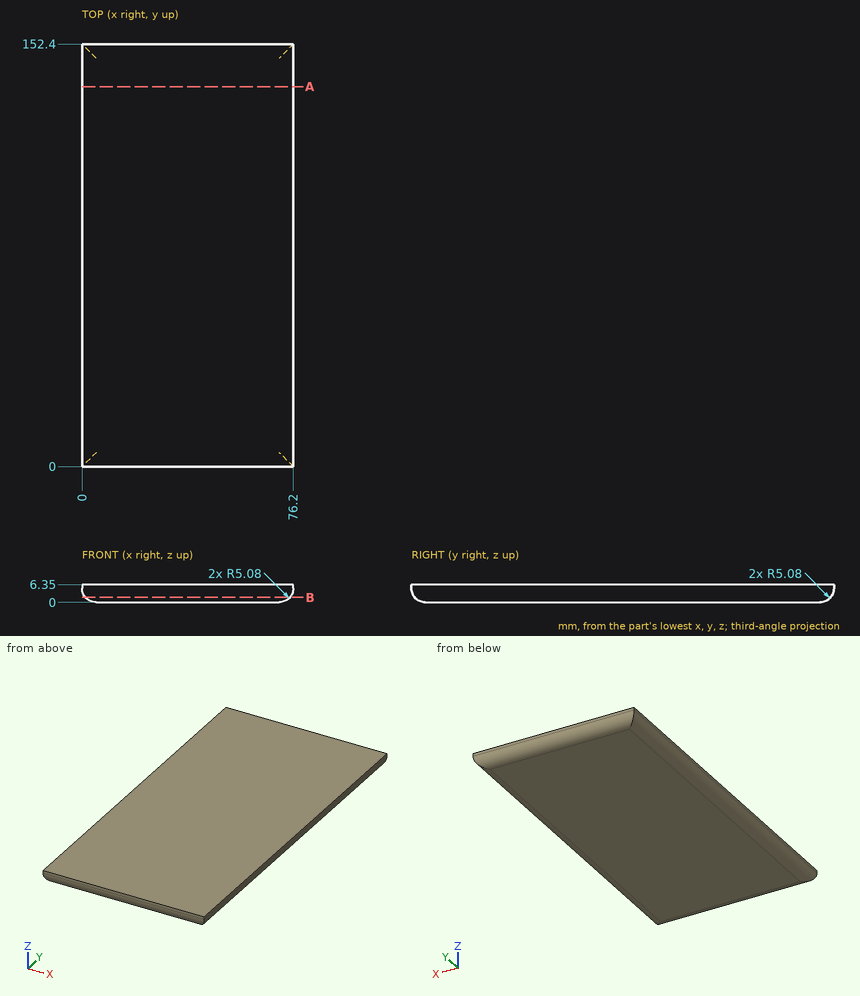
Source: three-view drawing plus pictorial views. Frame: mm from the lowest corner of the part. Give positions to 0.01 mm unless a question says otherwise; leave off trailing zeros. Write each loop counter-clockwise with the first axis right and the second up, starting at its lowest first coordinate (ties: lowest second). Pieces come first, ordered by that corner, then holes. Notation, with made-up numbers: (10.25, -36.75) -> (61.25, -36.75) arc R16 cw to (61.25, -27.75) -> close; hole circle Ø8 at (22, 23). An arc over 180 degrees is marked (long way). Answer in a Markdown table with one row per item.
(1) Pin query (flat end, axial travel): pin 1 (8 mm diameter, centred on x = 8.5, y = 16.5, fed in from -Z); pin 2 (1.5 mm diameter, centred on x = 56.5, z = 4, fed in from -Y). Return the tip coordinate at first contact, or that it passes through.
Answers below:
| item | result |
|---|---|
| pin 1 | z = 0 |
| pin 2 | y = 0.01 |
(2) Section query B-B on z = 1.75. Return loops of the section in (x, y), then the cut area to 3 significant figures.
Answers below:
| item | result |
|---|---|
| outline | (1.24, 1.24) -> (74.96, 1.24) -> (74.96, 151.16) -> (1.24, 151.16) -> close |
| area | 11,100 mm^2 |
(3) Section query A-A on y = 137. Return loops of the section in (x, z), then the cut area to 3 significant figures.
Answers below:
| item | result |
|---|---|
| outline | (0, 5.08) arc R5.08 ccw to (5.08, 0) -> (71.12, 0) arc R5.08 ccw to (76.2, 5.08) -> (76.2, 6.35) -> (0, 6.35) -> close |
| area | 473 mm^2 |
(4) Ray query, line 1 along X through (y, z) = (51.5, 4.5); line 2 along X through (y, z) = (35, 2.5); line 3 along Y through (x, z) = (48.5, 2). Return the intervals inside material, ascending. Write a range as [from, to].
Answers below:
| item | result |
|---|---|
| line 1 | [0.03, 76.17] |
| line 2 | [0.7, 75.5] |
| line 3 | [1.04, 151.36] |
